```python
from build123d import *

# Parameters (mm, degrees)
SKETCH1_R           = 1.537908455
BOSS_EXTRUDE1_DEPTH = 4
SKETCH2_R           = 20.698021895
SKETCH2_R_2         = 20.1
CUT_EXTRUDE1_DEPTH  = 1
SKETCH3_R           = 12.92497531
BOSS_EXTRUDE2_DEPTH = 0.5
SKETCH4_R           = 18.103513597
BOSS_EXTRUDE3_DEPTH = 6
FILLET1_R           = 1
BOSS_EXTRUDE4_DEPTH = 3
SCALE2_SCALE        = 0.5
SCALE3_SCALE        = 0.5


with BuildPart() as part:
    # Sketch1 → Boss-Extrude1 (new body)
    with BuildSketch(Plane.XY):
        with BuildLine():
            ThreePointArc((-17.85861924, -13.874920024), (0, -22.615120756), (17.85861924, -13.874920024))
            ThreePointArc((17.85861924, -13.874920024), (18.815427461, -12.936233048), (19.987223835, -12.285457765))
            add(Edge.make_bspline(
                [(19.987223835, -12.285457765), (51.427576939, 0), (19.987223835, 12.285457765)],
                knots=[5.385493495, 5.385493495, 5.385493495, 7.180877119, 7.180877119, 7.180877119], degree=2, weights=[1, 0.623416377, 1]))
            ThreePointArc((19.987223835, 12.285457765), (18.815427461, 12.936233048), (17.85861924, 13.874920024))
            ThreePointArc((17.85861924, 13.874920024), (0, 22.615120756), (-17.85861924, 13.874920024))
            ThreePointArc((-17.85861924, 13.874920024), (-18.815427461, 12.936233048), (-19.987223835, 12.285457765))
            add(Edge.make_bspline(
                [(-19.987223835, 12.285457765), (-51.427576939, 0), (-19.987223835, -12.285457765)],
                knots=[2.243900842, 2.243900842, 2.243900842, 4.039284465, 4.039284465, 4.039284465], degree=2, weights=[1, 0.623416377, 1]))
            ThreePointArc((-19.987223835, -12.285457765), (-18.815427461, -12.936233048), (-17.85861924, -13.874920024))
        make_face()
        with Locations((-29.809246855, 0)):
            Circle(SKETCH1_R, mode=Mode.SUBTRACT)
        with Locations((29.809246855, 0.098164369)):
            Circle(SKETCH1_R, mode=Mode.SUBTRACT)
    extrude(amount=BOSS_EXTRUDE1_DEPTH)

    # Sketch2 → Cut-Extrude1 (cut)
    with BuildSketch(Plane(origin=(0, 0, 0), x_dir=(-1, 0, 0), z_dir=(0, 0, -1))):
        Circle(SKETCH2_R)
        Circle(SKETCH2_R_2, mode=Mode.SUBTRACT)
    extrude(amount=-CUT_EXTRUDE1_DEPTH, mode=Mode.SUBTRACT)

    # Sketch3 → Boss-Extrude2 (add)
    with BuildSketch(Plane(origin=(0, 0, 0), x_dir=(-1, 0, 0), z_dir=(0, 0, -1))):
        Circle(SKETCH3_R)
    extrude(amount=BOSS_EXTRUDE2_DEPTH)

    # Sketch4 → Boss-Extrude3 (add)
    with BuildSketch(Plane(origin=(0, 0, -0.5), x_dir=(-1, 0, 0), z_dir=(0, 0, -1))):
        Circle(SKETCH4_R)
    extrude(amount=BOSS_EXTRUDE3_DEPTH)

    # Fillet1
    fillet1_edges = [part.edges().sort_by_distance(p)[0] for p in [
        (18.103513597, 0, -6.5),
    ]]
    fillet(fillet1_edges, radius=FILLET1_R)

    # Sketch5 → Boss-Extrude4 (add)
    with BuildSketch(Plane(origin=(0, 0, -6.5), x_dir=(-1, 0, 0), z_dir=(0, 0, -1))):
        with BuildLine():
            Line((-4.025670138, 1.472465542), (-17.702307957, 1.472465542))
            Line((-17.702307957, 1.472465542), (-18.467666717, 0.707106781))
            ThreePointArc((-18.467666717, 0.707106781), (-18.760559936, 0), (-18.467666717, -0.707106781))
            Line((-18.467666717, -0.707106781), (-17.702307957, -1.472465542))
            Line((-17.702307957, -1.472465542), (-4.025670138, -1.472465542))
            ThreePointArc((-4.025670138, -1.472465542), (0, -4.286510799), (4.025670138, -1.472465542))
            Line((4.025670138, -1.472465542), (17.636865044, -1.472465542))
            Line((17.636865044, -1.472465542), (18.402223804, -0.707106781))
            ThreePointArc((18.402223804, -0.707106781), (18.695117023, 0), (18.402223804, 0.707106781))
            Line((18.402223804, 0.707106781), (17.636865044, 1.472465542))
            Line((17.636865044, 1.472465542), (4.025670138, 1.472465542))
            ThreePointArc((4.025670138, 1.472465542), (0, 4.286510799), (-4.025670138, 1.472465542))
        make_face()
    extrude(amount=BOSS_EXTRUDE4_DEPTH)


with BuildPart() as part_1:
    # Scale2: scaled about (0, 0, 0)
    add(part.part.scale(SCALE2_SCALE))


with BuildPart() as part_2:
    # Scale3: scaled about (0, 0, 0)
    add(part_1.part.scale(SCALE3_SCALE))


solid = part_2.part
```
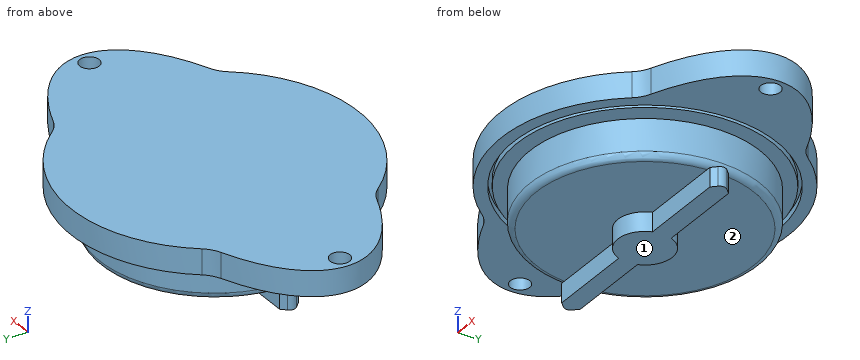
Verification items for the finished model (mm, model axes). Face numbers are marked on the shaded views. A direction names the side the tool comes from. Round coordinates to 2 decimals unless told otherwise and drop trailing zeros. Write each loop counter-clockwise with the first axis right and the second up, starting at its lowest first coordinate (ties: lowest second). Pieces come first, ordered by that corner, then holes.
1. Section check C-C on z = -0.3. Enter the section's corners in (x, y).
2. Gauge pin test, flat ends, axial feed: P1, Ø3, axis at x = 2, y = -3, coming from the -Z side (3 decimals); P2, Ø3, axis at x = 0.5, y = 2, coming from the -Z side (3 decimals); P3, Ø1, axis at y = 0, z = -1.5, coming from the -X side; P4, Ø2, axis at x = -0.5, z = -2, coming from the +Y side. Record the tip position at first contact, or that the pin passes through.
3. Section check B-B on z = 0.75. State how many separate pieces and enclosed holes the cut face has, plus the area to 3 significant figures.
4. Scan lines: L1, parallel to Z at x = -5.5, y = -2.5; L2, parallel to Y at x = -1.5, z = -2.15; L3, parallel to Y at x = 4.5, z = 0.2. Record each from-to range of solid material in increasing order.
5. Access from +Z, -Z, +X, -X, +Y, -Y to the whole of each face (thin tool, end or side, straight path). Record for the marked faces 1 and 2.
Answer:
1. outline: circle Ø9.05 at (0, 0)
2. P1: stops at z = -1.625
2. P2: stops at z = -2.375
2. P3: stops at x = -4.67
2. P4: stops at y = 4.53
3. separate pieces: 1
3. enclosed holes: 2
3. area: 121 mm2
4. L1: z = 0 to 1
4. L2: y = -0.37 to 0.37
4. L3: y = -3.43 to -2.55, -2.24 to 2.24, 2.55 to 3.43
5. face 1: -Z, +X, -X, +Y, -Y
5. face 2: -Z, +Y
